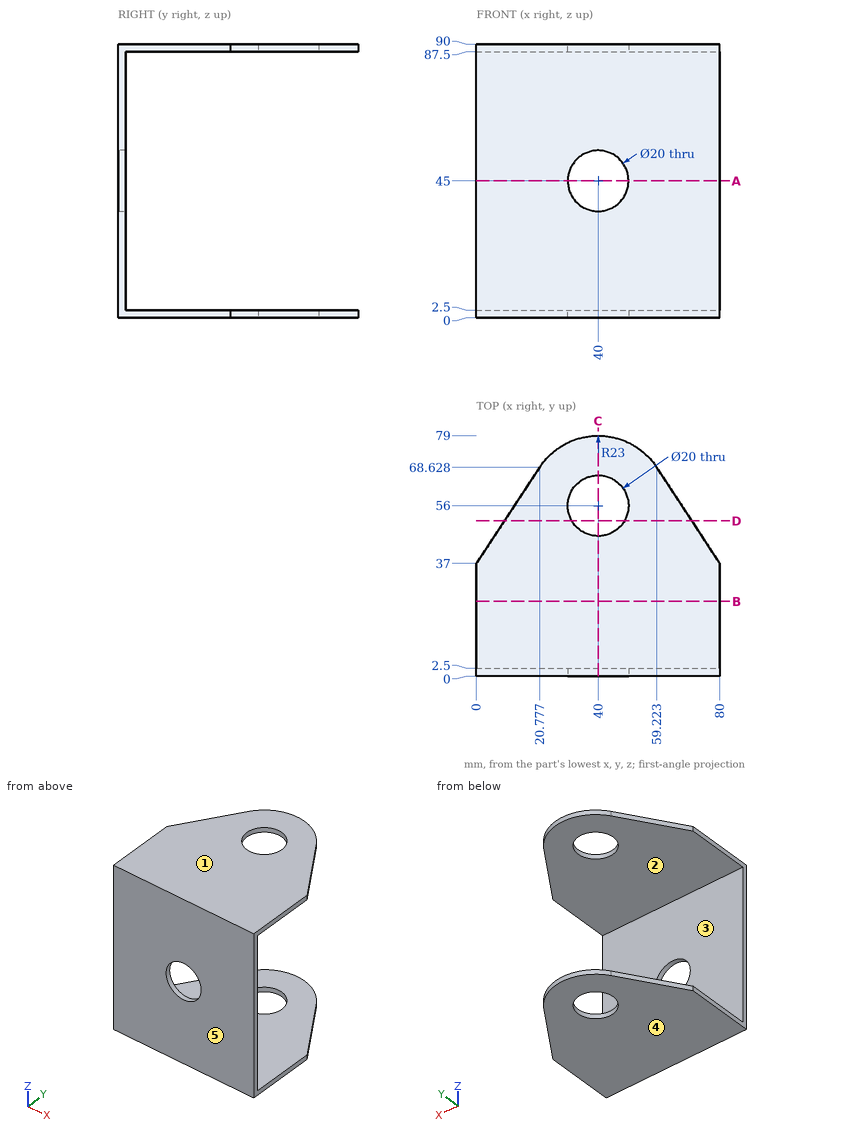
Drawing for the job (mm, zero at the part's lowest x, y, z). A direction names the side the tool comes from. Round coordinates to 2 decimals unless told otherwise and drop trailing zeros. Write each loop counter-clockwise with the first axis right and the second up, starting at its lowest first coordinate (ties: lowest second). Pieces come first, ordered by that corner, then holes. Notation, with made-up numbers: (50.5, 17) - (58.5, 17) arc R7 ccw to (58.5, 21) - close; hole circle Ø7 at (66, 52.25). An arc over 180 degrees is marked (long way). Write item = value, one per line. Start each with the question number.
Q1. Mould opens along Z. For the marked faces 3, 4 and 5 say: pulls with the +Z half, pulls with the -Z half, needs draft (parallel to the pull), parting line crosses it, or undercut.
Q2. Band-saw the part on C-C (x = 40). Give the cut face in (y, z).
Q3. Band-saw the part on D-D (y = 51). Give the cut face in (x, z).
Q4. Drop a flat-ended pin along its axis: pin 1 (1.5 mm diameter, centred on x = 20.5, z = 34.5, fed in from +Y). Give the stop position or say it passes through.
Q5. Band-saw the part on B-B (y = 24.5). Give the cut face in (x, z).
Q6. Probe L1, parallel to Z at x = 13.5, y = 25; L2, parallel to Y at x = 40, z = 88.75; L3, parallel to Y at x = 45, z = 70.5. List the from-to ranges inside material, lowest first. Write a range as from..to.
Q7. Which spindle directions (+Z, -Z, +X, -X, +Y, -Y) get a long thin tool onto all of the face, cutting with end or side? Do the marked faces 1 and 2. Say none if no direction does.
Q8. Band-saw the part on A-A (z = 45). Give the cut face in (x, y).
Answers below:
q1.face_3 = undercut
q1.face_4 = pulls with the -Z half
q1.face_5 = needs draft
q2.outline = (0, 0) - (46, 0) - (46, 2.5) - (2.5, 2.5) - (2.5, 35) - (0, 35) - close; (0, 55) - (2.5, 55) - (2.5, 87.5) - (46, 87.5) - (46, 90) - (0, 90) - close; (66, 0) - (79, 0) - (79, 2.5) - (66, 2.5) - close; (66, 87.5) - (79, 87.5) - (79, 90) - (66, 90) - close
q3.outline = (9.2, 0) - (31.34, 0) - (31.34, 2.5) - (9.2, 2.5) - close; (9.2, 87.5) - (31.34, 87.5) - (31.34, 90) - (9.2, 90) - close; (48.66, 0) - (70.8, 0) - (70.8, 2.5) - (48.66, 2.5) - close; (48.66, 87.5) - (70.8, 87.5) - (70.8, 90) - (48.66, 90) - close
q4.pin_1 = 2.5
q5.outline = (0, 0) - (80, 0) - (80, 2.5) - (0, 2.5) - close; (0, 87.5) - (80, 87.5) - (80, 90) - (0, 90) - close
q6.L1 = 0..2.5, 87.5..90
q6.L2 = 0..46, 66..79
q6.L3 = 0..2.5
q7.face_1 = +Z, +X, -X, +Y, -Y
q7.face_2 = +X, -X, +Y
q8.outline = (0, 0) - (30, 0) - (30, 2.5) - (0, 2.5) - close; (50, 0) - (80, 0) - (80, 2.5) - (50, 2.5) - close
